For this review, take the finished solid that the model builds, in its own axes (mm). Face numbers are marked on the shaded views. A direction names the side the tool comes from. Give positions to 0.01 mm unless a question says otherwise; leave off trailing zeros. Order: outer loops, then holes, each group sorted by start corner. A loop starts at its lowest first (then second) coordinate and runs counter-clockwise, first axis right, second up.
Item 1: Consider section A-A (x = 185). Give the boundary of the cut face in (y, z).
Item 2: For probe 1 along Y at (x, z) = (34.5, 8.5); probe 2 along X at (y, z) = (11.25, 2.75); probe 3 along Y at (x, z) = (126.5, 3), list the stretches that pass through material, from the lowest coordinate up.
Item 3: Consider section C-C (x = 135). Give the boundary of the cut face in (y, z).
Item 4: Machinability: for the marked faces 1 and 2, which of the approach directions +Z, -Z, +X, -X, +Y, -Y give a long, thin tool a straight path to every point of the face, cutting with its end or side? Answer none if there is none.
Item 5: Consider section B-B (y = 10). Give the boundary of the cut face in (x, z), plus the area to 3 significant figures.
```python
from build123d import *

# Parameters (mm, degrees)
F1_DEPTH = 10
F3_DEPTH = 200.001
F5_DEPTH = 10


with BuildPart() as f1:
    # F0 (on Top) → F1 (new body)
    with BuildSketch(Plane.XY):
        with BuildLine():
            ThreePointArc((20, 20), (15, 15), (10, 20))
            ThreePointArc((10, 20), (5, 25), (0, 20))
            Line((0, 20), (0, 0))
            Line((0, 0), (200, 0))
            Line((200, 0), (200, 20))
            ThreePointArc((200, 20), (195, 15), (190, 20))
            ThreePointArc((190, 20), (185, 25), (180, 20))
            ThreePointArc((180, 20), (175, 15), (170, 20))
            ThreePointArc((170, 20), (165, 25), (160, 20))
            ThreePointArc((160, 20), (155, 15), (150, 20))
            ThreePointArc((150, 20), (145, 25), (140, 20))
            ThreePointArc((140, 20), (135, 15), (130, 20))
            ThreePointArc((130, 20), (125, 25), (120, 20))
            ThreePointArc((120, 20), (115, 15), (110, 20))
            ThreePointArc((110, 20), (105, 25), (100, 20))
            ThreePointArc((100, 20), (95, 15), (90, 20))
            ThreePointArc((90, 20), (85, 25), (80, 20))
            ThreePointArc((80, 20), (75, 15), (70, 20))
            ThreePointArc((70, 20), (65, 25), (60, 20))
            ThreePointArc((60, 20), (55, 15), (50, 20))
            ThreePointArc((50, 20), (45, 25), (40, 20))
            ThreePointArc((40, 20), (35, 15), (30, 20))
            ThreePointArc((30, 20), (25, 25), (20, 20))
        make_face()
    extrude(amount=F1_DEPTH)

    # F2 (on face) → F3 (cut, through all)
    with BuildSketch(Plane(origin=(0, 0, 0), x_dir=(0, -1, 0), z_dir=(-1, 0, 0))):
        Polygon((0, 2), (0, 8), (-5.196152, 5), align=None)
    extrude(amount=-F3_DEPTH, mode=Mode.SUBTRACT)

    # F4 (on face) → F5 (cut, through all)
    with BuildSketch(Plane.XY.offset(10)):
        with BuildLine():
            ThreePointArc((8, 17.196152), (5, 20.196152), (2, 17.196152))
            Line((2, 17.196152), (2, 8.196152))
            Line((2, 8.196152), (14.824948, 8.196152))
            Line((14.824948, 8.196152), (28, 8.196152))
            Line((28, 8.196152), (198, 8.196152))
            Line((198, 8.196152), (198, 13.081795))
            ThreePointArc((198, 13.081795), (192.130857, 13.026509), (188, 17.196152))
            ThreePointArc((188, 17.196152), (185, 20.196152), (182, 17.196152))
            ThreePointArc((182, 17.196152), (175, 12.459339), (168, 17.196152))
            ThreePointArc((168, 17.196152), (165, 20.196152), (162, 17.196152))
            ThreePointArc((162, 17.196152), (155, 12.459339), (148, 17.196152))
            ThreePointArc((148, 17.196152), (145, 20.196152), (142, 17.196152))
            ThreePointArc((142, 17.196152), (135, 12.459339), (128, 17.196152))
            ThreePointArc((128, 17.196152), (125, 20.196152), (122, 17.196152))
            ThreePointArc((122, 17.196152), (115, 12.459339), (108, 17.196152))
            ThreePointArc((108, 17.196152), (105, 20.196152), (102, 17.196152))
            ThreePointArc((102, 17.196152), (95, 12.459339), (88, 17.196152))
            ThreePointArc((88, 17.196152), (85, 20.196152), (82, 17.196152))
            ThreePointArc((82, 17.196152), (75, 12.459339), (68, 17.196152))
            ThreePointArc((68, 17.196152), (65, 20.196152), (62, 17.196152))
            ThreePointArc((62, 17.196152), (55, 12.459339), (48, 17.196152))
            ThreePointArc((48, 17.196152), (45, 20.196152), (42, 17.196152))
            ThreePointArc((42, 17.196152), (35, 12.459339), (28, 17.196152))
            ThreePointArc((28, 17.196152), (25, 20.196152), (22, 17.196152))
            ThreePointArc((22, 17.196152), (15, 12.459339), (8, 17.196152))
        make_face()
    extrude(amount=-F5_DEPTH, mode=Mode.SUBTRACT)


solid = f1.part
```
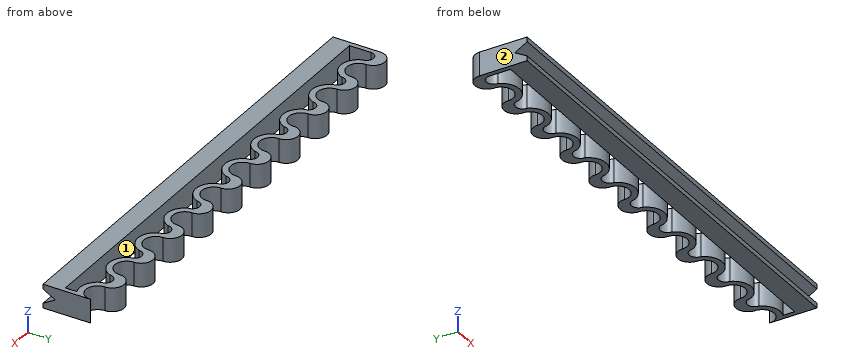
Resolved:
1. outline: (0, 0) - (8.2, 0) - (8.2, 10) - (0, 10) - (0, 8) - (5.2, 5) - (0, 2) - close; (20.2, 0) - (25, 0) - (25, 10) - (20.2, 10) - close
2. probe 1: y = 0 to 8.2, 12.48 to 15.03
2. probe 2: x = 0 to 2, 198 to 200
2. probe 3: y = 1.73 to 8.2, 19.79 to 24.77
3. outline: (0, 0) - (8.2, 0) - (8.2, 10) - (0, 10) - (0, 8) - (5.2, 5) - (0, 2) - close; (12.46, 0) - (15, 0) - (15, 10) - (12.46, 10) - close
4. face 1: +Z, -Z
4. face 2: +Z, -Z, -X, +Y, -Y
5. outline: (0, 0) - (2, 0) - (2, 10) - (0, 10) - close; (198, 0) - (200, 0) - (200, 10) - (198, 10) - close
5. area: 40.0 mm2
